Design review of the part shown in the three views and the two pictorial views. Dimensions are in mm from the part's minimum x, y and z. Give positions to 0.01 mm unless a question says otherwise; leave off trailing zeros. Order: outer loops, then holes, each group sorted by start corner. A loop starts at its lowest first (then second) coordinate and runs counter-clockwise, first axis right, second up.
Item 1: For probe 1 along Z at (x, y) = (3.5, 2.9); probe 2 along Z at (x, y) = (1.1, 3); probe 3 along Y at (x, z) = (3.85, 26.75) (1 decimal), list the stretches that pass through material, from the lowest coordinate up.
Item 2: For P1, Ø3, axis at y = 3.5, z = 21.5, coming from the +X side; P2, Ø1.5, axis at x = 1, z = 23, coming from the -Y side; P3, Ø3, axis at x = 4.5, y = 4.5, coming from the -Z side (1 decimal), all flat-tipped, find the tip position at first contact; note any pin that passes through.
Item 3: Consider section A-A (x = 2.7). Give the boundary of the cut face in (y, z).
Item 4: The part is to be moulded in two halves that separate along Y. For the marked faces 1 and 2, say which applies: released by +Y, released by -Y, zero draft, split by the parting line, or undercut.
Item 5: Consider section B-B (z = 25.5). Give the boundary of the cut face in (x, y).
Item 6: Consider section C-C (z = 22.5). Give the boundary of the cut face in (x, y).
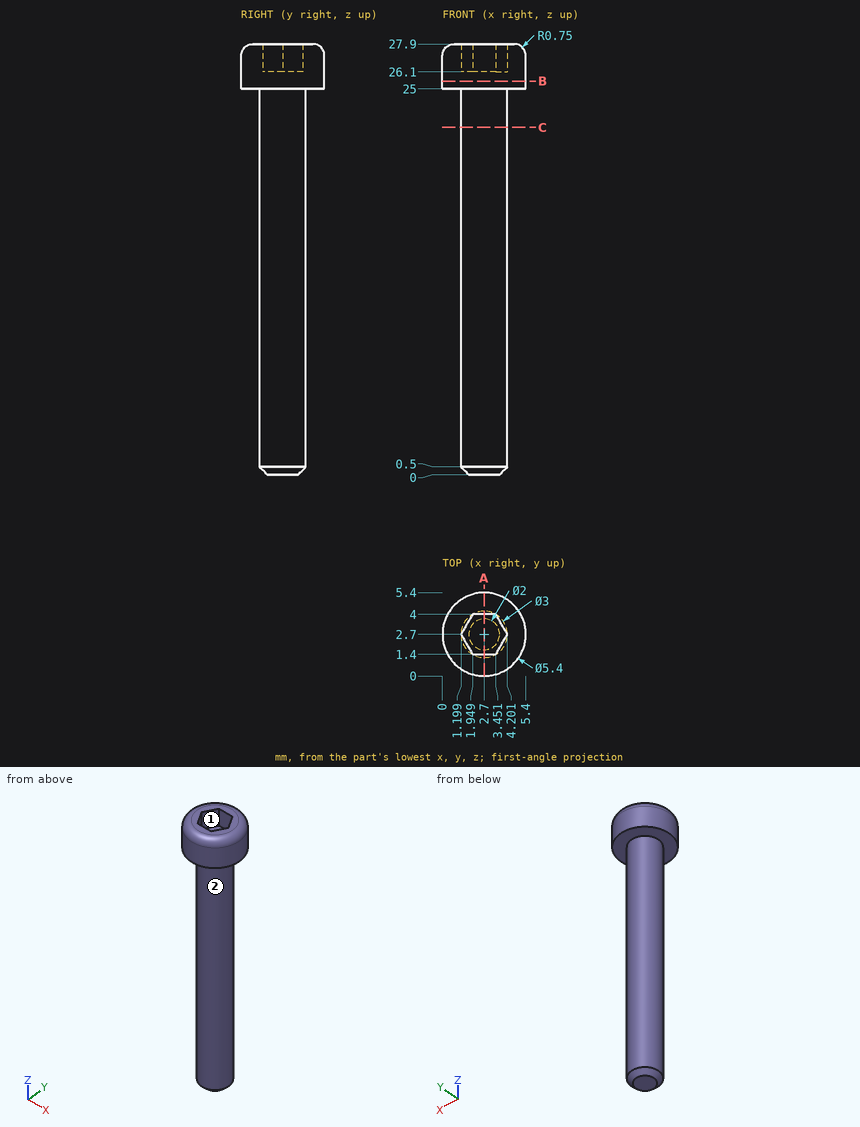
Resolved:
1. probe 1: z = 0 to 26.1
1. probe 2: z = 25 to 27.9
1. probe 3: y = 0.3 to 2.1, 3.3 to 5.1
2. P1: stops at x = 4.2
2. P2: stops at y = 1.54
2. P3: stops at z = 0
3. outline: (0, 25) - (1.2, 25) - (1.2, 0.5) - (1.7, 0) - (3.7, 0) - (4.2, 0.5) - (4.2, 25) - (5.4, 25) - (5.4, 27.15) arc R0.75 ccw to (4.65, 27.9) - (4, 27.9) - (4, 26.1) - (1.4, 26.1) - (1.4, 27.9) - (0.75, 27.9) arc R0.75 ccw to (0, 27.15) - close
4. face 1: undercut
4. face 2: split by the parting line
5. outline: circle Ø5.4 at (2.7, 2.7)
6. outline: circle Ø3 at (2.7, 2.7)
